from build123d import *

# Parameters (mm, degrees)
SKETCH1_W           = 12.7
SKETCH1_H           = 12.7
BOSS_EXTRUDE1_DEPTH = 2.54
FILLET1_R           = 0.635
SHELL1_START        = 0.635
SHELL1_OUTLINE_W    = 1.905
SHELL1_OUTLINE_H    = 11.43
SHELL1_DEPTH        = 11.43
SKETCH2_R           = 2.54
BOSS_EXTRUDE2_DEPTH = 1.905
SKETCH3_W           = 2.157371795
SKETCH3_H           = 0.529166666
SKETCH3_H_2         = 0.529166667
BOSS_EXTRUDE3_DEPTH = 0.00254


# Read off the part's stored shape, not the designer's step: Shell1
with BuildPart() as part:
    # Sketch1 → Boss-Extrude1 (new body)
    with BuildSketch(Plane(origin=(0, 0, 0), x_dir=(1, 0, 0), z_dir=(0, 1, 0))):
        with Locations((6.35, 6.35)):
            Rectangle(SKETCH1_W, SKETCH1_H)
    extrude(amount=BOSS_EXTRUDE1_DEPTH)

    # Fillet1
    fillet1_edges = [part.edges().sort_by_distance(p)[0] for p in [
        (0, 1.27, -12.7),
        (12.7, 1.27, -12.7),
        (12.7, 1.27, 0),
        (0, 1.27, 0),
    ]]
    fillet(fillet1_edges, radius=FILLET1_R)

    # Shell1 outline → Shell1 (cut)
    with BuildSketch(Plane.YZ.offset(SHELL1_START)):
        with Locations((0.9525, -6.35)):
            Rectangle(SHELL1_OUTLINE_W, SHELL1_OUTLINE_H)
    extrude(amount=SHELL1_DEPTH, mode=Mode.SUBTRACT)

    # Sketch2 → Boss-Extrude2 (add)
    with BuildSketch(Plane(origin=(0, 1.905, 0), x_dir=(-1, 0, 0), z_dir=(0, -1, 0))):
        with Locations(Location((-6.35, 6.35, 0), (0, 0, 270))):
            Circle(SKETCH2_R)
    extrude(amount=BOSS_EXTRUDE2_DEPTH)

    # Sketch3 → Boss-Extrude3 (add)
    with BuildSketch(Plane(origin=(0, 2.54, 0), x_dir=(1, 0, 0), z_dir=(0, 1, 0))):
        Polygon((6.239933333, 8.903025641), (6.239933333, 9.676423077), (6.7691, 9.676423077), (6.7691, 8.903025641), (7.583202564, 8.903025641), (7.583202564, 8.373858974), (6.7691, 8.373858974), (6.7691, 7.600461538), (6.239933333, 7.600461538), (6.239933333, 8.373858974), (5.425830769, 8.373858974), (5.425830769, 8.903025641), align=None)
        with Locations((6.529916667, 4.554903846)):
            Rectangle(SKETCH3_W, SKETCH3_H)
        with Locations((6.529916667, 3.659391026)):
            Rectangle(SKETCH3_W, SKETCH3_H_2)
    extrude(amount=BOSS_EXTRUDE3_DEPTH)


solid = part.part
Geometry: final body of the model. Coordinates: model frame, mm. A direction names the side the tool comes from. Round coordinates to 2 decimals unless told otherwise and drop trailing zeros. Write each loop counter-clockwise with the first axis right and the second up, starting at its lowest first coordinate (ties: lowest second). Pieces come first, ordered by that corner, then holes. Notation, with made-up numbers: M 72,-38 L 76,-38 A16 ccw 76,-14 Z; hole C 59,21 d10. An arc over 180 degrees is marked long. Write item = value, one per line.
Item 1: Material intervals for line 1 along Z through (x, y) = (6.5, 0.5) (3 decimals); line 2 along X through (y, z) = (1.55, -6.25) (3 decimals); line 3 along X through (y, z) = (1.1, -1.5) (3 decimals), sorted ascending. Write a range as [from, to].
Findings:
line_1 = [-12.7, -12.065], [-8.886, -3.814], [-0.635, 0]
line_2 = [0, 0.635], [3.812, 8.888], [12.065, 12.7]
line_3 = [0, 0.635], [12.065, 12.7]
Item 2: Section query C-C on x = 2. Return loops of the section in (y, z) (3 decimals).
Findings:
outline = M 0,-12.7 L 2.54,-12.7 L 2.54,0 L 0,0 L 0,-0.635 L 1.905,-0.635 L 1.905,-12.065 L 0,-12.065 Z
Item 3: Section query B-B on z = -10. Return loops of the section in (x, y) (3 decimals), then the cut area to 3 significant figures.
Findings:
outline = M 0,0 L 0.635,0 L 0.635,1.905 L 12.065,1.905 L 12.065,0 L 12.7,0 L 12.7,2.54 L 0,2.54 Z
area = 10.5 mm^2
Item 4: Pull-direction query (X, two-part tool) for faces 3 (the face through (8.83, 0.97, -6.9)), 4 (the face through (0, 1, -6)), 5 (the face through (6, 0, -6)), 6 (the face through (12.7, 1, -6)); classes: pulls with the +X half, pulls with the -X half, needs draft (parallel to the pull), parting line crosses it, or undercut.
Findings:
face_3 = undercut
face_4 = pulls with the -X half
face_5 = needs draft
face_6 = pulls with the +X half
Item 5: Section query A-A on y = 1.25. Return loops of the section in (x, z) (3 decimals), then the cut area to 3 significant figures.
Findings:
outline = M 0,-12.065 A0.635 ccw 0.635,-12.7 L 12.065,-12.7 A0.635 ccw 12.7,-12.065 L 12.7,-0.635 A0.635 ccw 12.065,0 L 0.635,0 A0.635 ccw 0,-0.635 Z; C 6.35,-6.35 d5.08; hole M 0.635,-12.065 L 12.065,-12.065 L 12.065,-0.635 L 0.635,-0.635 Z
area = 50.6 mm^2
Item 6: Section query D-D on z = -6. Return loops of the section in (x, y) (3 decimals), then the cut area to 3 significant figures.
Findings:
outline = M 0,0 L 0.635,0 L 0.635,1.905 L 3.834,1.905 L 3.834,0 L 8.866,0 L 8.866,1.905 L 12.065,1.905 L 12.065,0 L 12.7,0 L 12.7,2.54 L 0,2.54 Z
area = 20.1 mm^2
Item 7: Access query for faces 1 (the face through (6, 1, -12.7)), 2 (the face through (0.635, 1, -6)). Directions: +Z, -Z, +X, -X, +Y, -Y. A direction counts if a zero-diameter tool reaches every point of the face in a straight line with its end or side. Return the directions, or none.
Findings:
face_1 = -Z, +X, -X, +Y, -Y
face_2 = -Y
